Verification items for this drawing (mm, ordinates from the low corner). Coordinates: 2 decimals unless noted, no trailing zeros. Write each loop counter-clockwise with the first axis right and the second up, starting at its lowest first coordinate (ties: lowest second). Pieces come first, ordered by that corner, then holes. Notation, with made-up numbers: (-7.75, 18.5) -> (22.25, 18.5) arc R24 cw to (22.25, 28.5) -> close; hole circle Ø8 at (73.25, 40.5). An arc over 180 degrees is marked (long way). One line per item, written item: value. Start each with the question number.
1) Sectioned sample at D-D on x = 102.5. Enter the section's corners in (y, z) (3 decimals).
2) Sectioned sample at C-C on x = 75.5. Enter the section's corners in (y, z) (3 decimals).
3) Sectioned sample at A-A on z = 1.8. Enter the section's corners in (x, y) (3 decimals).
4) Gauge pin test, flat ends, axial feed: P1, Ø2.5, axis at x = 3.5, y = 2, coming from the +Z side; P2, Ø1, axis at x = 37.5, y = 23, coming from the +Z side; P3, Ø1.2, axis at x = 79.5, z = 1.5, coming from the -Y side (3 decimals); P4, Ø0.8, axis at y = 2, z = 1.5, coming from the -X side. Record the tip position at first contact, or that the pin passes through.
5) Sectioned sample at B-B on y = 12.75. Enter the section's corners in (x, z), plus the area to 3 significant figures.
6) Scan lines: line 1 along X through (y, z) = (19.75, 1.25); line 2 along Y through (x, z) = (42.5, 1.45) (3 decimals); line 3 along X through (y, z) = (10.5, 0.25). Record each from-to range of solid material in increasing order. Write a range as [from, to].
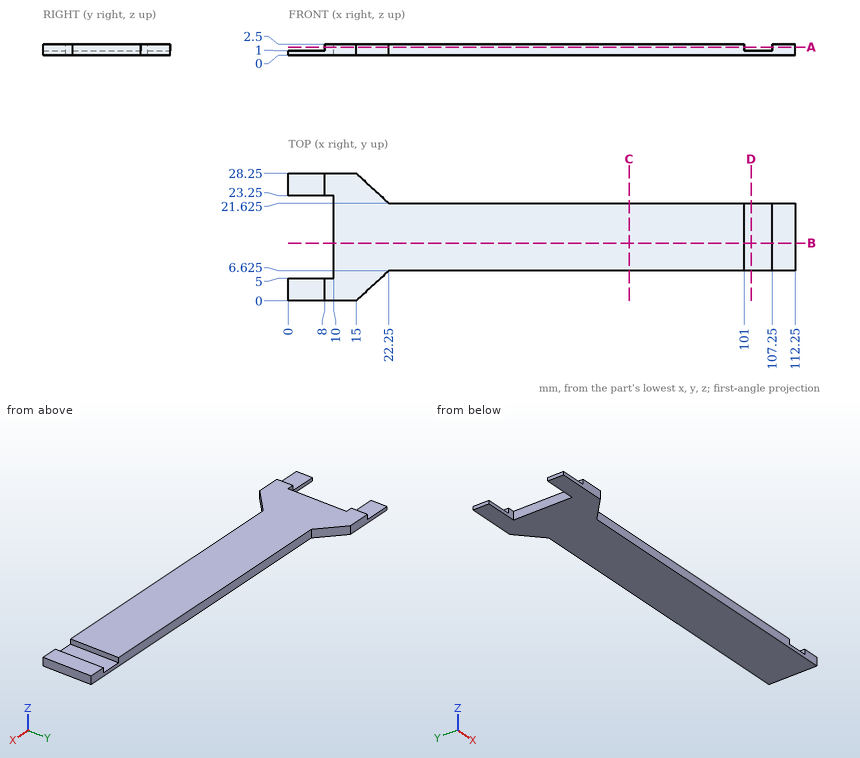
Answers:
1. outline: (6.625, 0) -> (21.625, 0) -> (21.625, 1) -> (6.625, 1) -> close
2. outline: (6.625, 0) -> (21.625, 0) -> (21.625, 2.5) -> (6.625, 2.5) -> close
3. outline: (8, 0) -> (15, 0) -> (22.25, 6.625) -> (101, 6.625) -> (101, 21.625) -> (22.25, 21.625) -> (15, 28.25) -> (8, 28.25) -> (8, 23.25) -> (10, 23.25) -> (10, 5) -> (8, 5) -> close; (107.25, 6.625) -> (112.25, 6.625) -> (112.25, 21.625) -> (107.25, 21.625) -> close
4. P1: stops at z = 1
4. P2: passes through
4. P3: stops at y = 6.625
4. P4: stops at x = 8
5. outline: (10, 0) -> (112.25, 0) -> (112.25, 2.5) -> (107.25, 2.5) -> (107.25, 1) -> (101, 1) -> (101, 2.5) -> (10, 2.5) -> close
5. area: 246 mm2
6. line 1: x = [10, 101], [107.25, 112.25]
6. line 2: y = [6.625, 21.625]
6. line 3: x = [10, 112.25]
